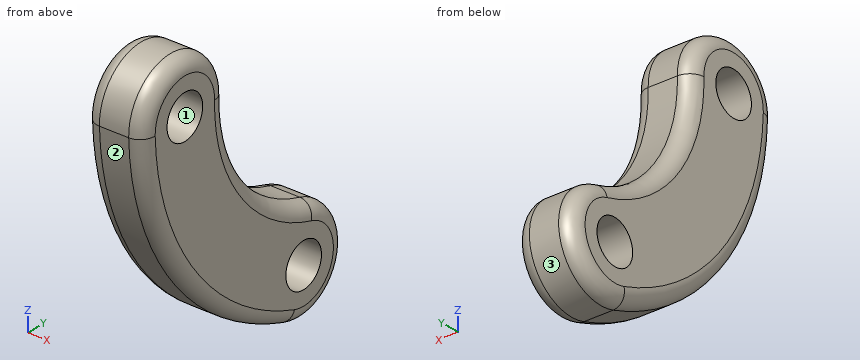
```python
from build123d import *

# Parameters (mm, degrees)
SKETCH1_R           = 15
BOSS_EXTRUDE1_DEPTH = 40
FILLET1_R           = 10


with BuildPart() as part:
    # Sketch1 → Boss-Extrude1 (new body)
    with BuildSketch(Plane(origin=(0, 0, 0), x_dir=(0, 0, -1), z_dir=(1, 0, 0))):
        with BuildLine():
            ThreePointArc((33.277008782, -10.846229138), (9.959027872, 33.553207952), (-33.805757942, 9.064807223))
            ThreePointArc((-33.805757942, 9.064807223), (-70.44161018, -45.071700409), (-132.694646831, -65.009266851))
            ThreePointArc((-132.694646831, -65.009266851), (-168.499781041, -100.12380247), (-132.447129149, -134.984160172))
            ThreePointArc((-132.447129149, -134.984160172), (-29.948243855, -99.130344454), (33.277008782, -10.846229138))
        make_face()
        Circle(SKETCH1_R, mode=Mode.SUBTRACT)
        with Locations((-133.5, -100)):
            Circle(SKETCH1_R, mode=Mode.SUBTRACT)
    extrude(amount=BOSS_EXTRUDE1_DEPTH)

    # Fillet1
    fillet1_edges = [part.edges().sort_by_distance(p)[0] for p in [
        (40, -45.071700409, 70.44161018),
        (40, -100.12380247, 168.499781041),
        (40, -99.130344454, 29.948243855),
        (0, -100.12380247, 168.499781041),
        (0, -45.071700409, 70.44161018),
        (0, 33.553207952, -9.959027872),
        (0, -99.130344454, 29.948243855),
        (40, 33.553207952, -9.959027872),
    ]]
    fillet(fillet1_edges, radius=FILLET1_R)


solid = part.part
```
Geometry: final body of the model. Coordinates: model frame, mm. Face numbers are marked on the shaded views. Round coordinates to 2 decimals unless told otherwise and drop trailing zeros. Loops run counter-clockwise (first coordinate to the right, second up) from the corner with the lowest first, then second, coordinate; pieces in that order, holes last. Notation, with made-up numbers: (5, 35) -> (58, 35) arc R7 ccw to (58, 43) -> close; hole circle Ø5 at (76.25, 84). An arc over 180 degrees is marked (long way). Use one line per item in the form item = value. Start each with the question number.
1) Section A-A on x = 16.5. Output: boundary loops of the cut face in (y, z).
2) First-contact query: P1, Ø6, axis at x = 12.5, z = 96.5, coming from the -Y side; P2, Ø6, axis at x = 34.5, z = -9, coming from the -Y side; P3, Ø6, axis at x = 15.5, y = -96, coming from the -Z side; P4, Ø24, axis at y = 0, z = 0, coming from the -X side. Flat tips, straight axial feed; report the tip coordinate or a pass-through.
3) Draft query along Z for the marked faces 1, 2 and 3. Return one class per face: released by +Z, released by -Z, zero draft, split by the parting line, or undercut.
4) Section B-B on x = 32.5. Output: boundary loops of the cut face in (y, z).
5) Line query: L1, parallel to Y at x = 28, z = 133.5; L2, parallel to Y at x = 9, z = 133; L3, parallel to Z at x = 24.5, y = 1. Output: solid intervals per line, ascending.
Response:
q1.outline = (-134.98, 132.45) arc R180 ccw to (-10.85, -33.28) arc R35 ccw (long way) to (9.06, 33.81) arc R100 cw to (-65.01, 132.69) arc R35 ccw (long way) to start; hole circle Ø30 at (-100, 133.5); hole circle Ø30 at (0, 0)
q2.P1 = -130.93
q2.P2 = -61.98
q2.P3 = 22.22
q2.P4 = through
q3.face_1 = undercut
q3.face_2 = released by -Z
q3.face_3 = split by the parting line
q4.outline = (-134.67, 132.46) arc R179.68 ccw to (-10.75, -32.98) arc R34.68 ccw (long way) to (8.98, 33.5) arc R100.32 cw to (-65.33, 132.7) arc R34.68 ccw (long way) to start; hole circle Ø30 at (-100, 133.5); hole circle Ø30 at (0, 0)
q5.L1 = -135 to -115, -85 to -65
q5.L2 = -134.95 to -114.99, -85.01 to -65.05
q5.L3 = -34.99 to -14.97, 14.97 to 36.34
